from build123d import *

# Parameters (mm, degrees)
F1_DEPTH = 19.05


with BuildPart() as f1:
    # F0 (on Front) → F1 (new body, symmetric)
    with BuildSketch(Plane.XZ):
        with BuildLine():
            Line((4.33175, 0), (3.33175, 0))
            ThreePointArc((3.33175, 0), (0, -3.33175), (-3.33175, 0))
            Line((-3.33175, 0), (-4.33175, 0))
            Line((-4.33175, 0), (-4.33175, -5.83175))
            Line((-4.33175, -5.83175), (4.33175, -5.83175))
            Line((4.33175, -5.83175), (4.33175, 0))
        make_face()
    extrude(amount=F1_DEPTH, both=True)


solid = f1.part
Here's how the part is built. I have some questions about the finished solid (model axes, mm). Round coordinates to 2 decimals unless told otherwise and drop trailing zeros. Loops run counter-clockwise (first coordinate to the right, second up) from the corner with the lowest first, then second, coordinate; pieces in that order, holes last. Notation, with made-up numbers: (-3.75, 29.5) -> (12.25, 29.5) arc R12 cw to (12.25, 52.5) -> close; hole circle Ø8 at (-15, 54.5). An arc over 180 degrees is marked (long way). Write each question's results on one line, items separated by ' | '.
(1) If we section it at D-D, the plane x = 2: List the corners of the cut face in (y, z) for me.
Worked answers:
outline: (-19.05, -5.83) -> (19.05, -5.83) -> (19.05, -2.66) -> (-19.05, -2.66) -> close
(2) If I drill on L1, parallel to X at y = 0, z = -2.15; L2, parallel to X at y = -3, z = -1.55; L3, parallel to Z at x = 0, y = 14, over which ranges is the centre line in solid material (lowest first)?
Worked answers:
L1: -4.33 to -2.55, 2.55 to 4.33 | L2: -4.33 to -2.95, 2.95 to 4.33 | L3: -5.83 to -3.33
(3) If we section it at A-A, the plane z = -2.4: List the corners of the cut face in (x, y) for me.
Worked answers:
outline: (-4.33, -19.05) -> (-2.31, -19.05) -> (-2.31, 19.05) -> (-4.33, 19.05) -> close; (2.31, -19.05) -> (4.33, -19.05) -> (4.33, 19.05) -> (2.31, 19.05) -> close
(4) We'd pull the mould along X, two halves only. Please class faces 1 (the face through (-4.332, 0, -3)), 2 (the face through (0.07, -0.27, -3.33)), 3 (the face through (0, 19.05, -4)), 4 (the face through (4.332, 0, -3)): released by +X, released by -X, zero draft, split by the parting line, or undercut.
Worked answers:
face 1: released by -X | face 2: undercut | face 3: zero draft | face 4: released by +X
(5) If we section it at C-C, the plane x = 0: List the corners of the cut face in (y, z) for me.
Worked answers:
outline: (-19.05, -5.83) -> (19.05, -5.83) -> (19.05, -3.33) -> (-19.05, -3.33) -> close
(6) If we section it at B-B, the plane y = 16: List the corners of the cut face in (x, z) for me, then the cut area to 3 significant figures.
Worked answers:
outline: (-4.33, -5.83) -> (4.33, -5.83) -> (4.33, 0) -> (3.33, 0) arc R3.33 cw to (-3.33, 0) -> (-4.33, 0) -> close | area: 33.1 mm2
